Source: CAD feature listing. Evaluate the final solid. Frame: model axes, mm. A direction names the side the tool comes from. Give positions to 0.01 mm unless a question says otherwise; leave off trailing zeros. Order: outer loops, then holes, each group sorted by start corner. A loop starts at its lowest first (then second) coordinate and runs counter-clockwise, first axis right, second up.
from build123d import *

# Parameters (mm, degrees)
SKETCH_1_W          = 5000
SKETCH_1_H          = 1500
EXTRUDE_1_DEPTH     = 30
EXTRUDE_2_DEPTH     = 1500
EXTRUDE_3_REACH     = 5218.234
EXTRUDE_4_REACH     = 5168.168
SKETCH_5_W          = 130
SKETCH_5_H          = 10
FILLET_2_R          = 80
SKETCH_6_R          = 30
CUT_EXTRUDE_1_DEPTH = 1355
SCALE_1_SCALE       = 0.345


with BuildPart() as part:
    # 草图1 → 凸台-拉伸1 (new body)
    with BuildSketch(Plane.XY):
        with Locations((2446.443283418, -722.784179357)):
            Rectangle(SKETCH_1_W, SKETCH_1_H)
    extrude(amount=EXTRUDE_1_DEPTH)

    # 草图3 → 凸台-拉伸2 (add)
    with BuildSketch(Plane(origin=(0, 27.215820643, 0), x_dir=(1, 0, 0), z_dir=(0, 1, 0))):
        Polygon((-53.556716582, 0), (21.443283418, 0), (21.443283418, 200), (-53.556716582, 200), (-53.556716582, 191), (12.443283418, 191), (12.443283418, 9), (-53.556716582, 9), align=None)
        Polygon((4946.443283418, 9), (4946.443283418, 0), (4871.443283418, 0), (4871.443283418, 200), (4946.443283418, 200), (4946.443283418, 191), (4880.443283418, 191), (4880.443283418, 9), align=None)
    extrude(amount=-EXTRUDE_2_DEPTH)

    # 凸台-拉伸3: up to this face of the body (flat: up to its plane)
    extrude_3_end = Plane(part.part.faces().sort_by_distance((-53.556716582, -722.784179357, 10.5))[0])
    # 草图4 → 凸台-拉伸3 (add, up to the picked face)
    with BuildSketch(Plane(origin=(4946.443283418, 0, 0), x_dir=(0, 0, -1), z_dir=(1, 0, 0)), mode=Mode.PRIVATE) as extrude_3_sk1:
        Polygon((200, 27.215820643), (0, 27.215820643), (0, -47.784179357), (9, -47.784179357), (9, 18.215820643), (191, 18.215820643), (191, -47.784179357), (200, -47.784179357), align=None)
    extrude_3_tool1 = split(extrude(extrude_3_sk1.sketch, amount=-EXTRUDE_3_REACH, mode=Mode.PRIVATE), bisect_by=extrude_3_end, keep=Keep.BOTH, mode=Mode.PRIVATE)
    # 草图4 → 凸台-拉伸3 (add, up to the picked face)
    with BuildSketch(Plane(origin=(4946.443283418, 0, 0), x_dir=(0, 0, -1), z_dir=(1, 0, 0)), mode=Mode.PRIVATE) as extrude_3_sk2:
        Polygon((9, -1397.784179357), (0, -1397.784179357), (0, -1472.784179357), (200, -1472.784179357), (200, -1397.784179357), (191, -1397.784179357), (191, -1463.784179357), (9, -1463.784179357), align=None)
    extrude_3_tool2 = split(extrude(extrude_3_sk2.sketch, amount=-EXTRUDE_3_REACH, mode=Mode.PRIVATE), bisect_by=extrude_3_end, keep=Keep.BOTH, mode=Mode.PRIVATE)
    add(extrude_3_tool1.solids().sort_by(Axis((4946.443283, 25.07982, -100), (-1, 0, 0)))[0])
    add(extrude_3_tool2.solids().sort_by(Axis((4946.443283, -1399.92018, -4.5), (-1, 0, 0)))[0])

    # 凸台-拉伸4: up to this face of the body (flat: up to its plane)
    extrude_4_end = Plane(part.part.faces().sort_by_distance((2446.443283418, -722.784179357, 0))[0])
    # 草图5 → 凸台-拉伸4 (add, up to the picked face)
    with BuildSketch(Plane(origin=(0, 0, -200), x_dir=(-1, 0, 0), z_dir=(0, 0, -1)), mode=Mode.PRIVATE) as extrude_4_sk1:
        with Locations((-86.443283418, -52.784179357)):
            Rectangle(SKETCH_5_W, SKETCH_5_H)
    extrude_4_tool1 = split(extrude(extrude_4_sk1.sketch, amount=-EXTRUDE_4_REACH, mode=Mode.PRIVATE), bisect_by=extrude_4_end, keep=Keep.BOTH, mode=Mode.PRIVATE)
    # 草图5 → 凸台-拉伸4 (add, up to the picked face)
    with BuildSketch(Plane(origin=(0, 0, -200), x_dir=(-1, 0, 0), z_dir=(0, 0, -1)), mode=Mode.PRIVATE) as extrude_4_sk2:
        with Locations((-86.443283418, -174.784179357)):
            Rectangle(SKETCH_5_W, SKETCH_5_H)
    extrude_4_tool2 = split(extrude(extrude_4_sk2.sketch, amount=-EXTRUDE_4_REACH, mode=Mode.PRIVATE), bisect_by=extrude_4_end, keep=Keep.BOTH, mode=Mode.PRIVATE)
    # 草图5 → 凸台-拉伸4 (add, up to the picked face)
    with BuildSketch(Plane(origin=(0, 0, -200), x_dir=(-1, 0, 0), z_dir=(0, 0, -1)), mode=Mode.PRIVATE) as extrude_4_sk3:
        with Locations((-86.443283418, -1270.784179357)):
            Rectangle(SKETCH_5_W, SKETCH_5_H)
    extrude_4_tool3 = split(extrude(extrude_4_sk3.sketch, amount=-EXTRUDE_4_REACH, mode=Mode.PRIVATE), bisect_by=extrude_4_end, keep=Keep.BOTH, mode=Mode.PRIVATE)
    # 草图5 → 凸台-拉伸4 (add, up to the picked face)
    with BuildSketch(Plane(origin=(0, 0, -200), x_dir=(-1, 0, 0), z_dir=(0, 0, -1)), mode=Mode.PRIVATE) as extrude_4_sk4:
        with Locations((-86.443283418, -1392.784179357)):
            Rectangle(SKETCH_5_W, SKETCH_5_H)
    extrude_4_tool4 = split(extrude(extrude_4_sk4.sketch, amount=-EXTRUDE_4_REACH, mode=Mode.PRIVATE), bisect_by=extrude_4_end, keep=Keep.BOTH, mode=Mode.PRIVATE)
    add(extrude_4_tool1.solids().sort_by(Axis((86.443283, -52.784179, -200), (0, 0, 1)))[0])
    add(extrude_4_tool2.solids().sort_by(Axis((86.443283, -174.784179, -200), (0, 0, 1)))[0])
    add(extrude_4_tool3.solids().sort_by(Axis((86.443283, -1270.784179, -200), (0, 0, 1)))[0])
    add(extrude_4_tool4.solids().sort_by(Axis((86.443283, -1392.784179, -200), (0, 0, 1)))[0])

    # 圆角2
    # the kernel refuses this fillet: 80 mm, written as the material it takes off along each edge
    with BuildSketch(Plane(origin=(151.443283418, -47.784179357, -200), x_dir=(-1, 0, 0), z_dir=(0, -1, 0))) as fillet_2_piece_1:
        with BuildLine():
            CenterArc((FILLET_2_R, -FILLET_2_R), FILLET_2_R, 90, 90)
            Line((0, -FILLET_2_R), (0, 0))
            Line((0, 0), (FILLET_2_R, 0))
        make_face()
    extrude(amount=210, mode=Mode.SUBTRACT)
    with BuildSketch(Plane(origin=(151.443283418, 30.215820643, -200), x_dir=(-1, 0, 0), z_dir=(0, -1, 0))) as fillet_2_piece_2_section:
        with BuildLine():
            CenterArc((FILLET_2_R, -FILLET_2_R), FILLET_2_R, 90, 90)
            Line((0, -FILLET_2_R), (0, 0))
            Line((0, 0), (FILLET_2_R, 0))
        make_face()
    fillet_2_piece_2 = extrude(amount=410, mode=Mode.PRIVATE)
    fillet_2_piece_2 = split(fillet_2_piece_2, bisect_by=Plane(origin=(123.199877996, -47.784179357, -195.897838893), z_dir=(0, -1, 0)), keep=Keep.TOP, mode=Mode.PRIVATE)
    add(fillet_2_piece_2, mode=Mode.SUBTRACT)
    with BuildSketch(Plane(origin=(151.443283418, -1065.784179357, -200), x_dir=(-1, 0, 0), z_dir=(0, -1, 0))) as fillet_2_piece_3_section:
        with BuildLine():
            CenterArc((FILLET_2_R, -FILLET_2_R), FILLET_2_R, 90, 90)
            Line((0, -FILLET_2_R), (0, 0))
            Line((0, 0), (FILLET_2_R, 0))
        make_face()
    fillet_2_piece_3 = extrude(amount=410, mode=Mode.PRIVATE)
    fillet_2_piece_3 = split(fillet_2_piece_3, bisect_by=Plane(origin=(123.199877996, -1397.784179357, -195.897838893), z_dir=(0, 1, 0)), keep=Keep.TOP, mode=Mode.PRIVATE)
    add(fillet_2_piece_3, mode=Mode.SUBTRACT)
    with BuildSketch(Plane(origin=(151.443283418, -1397.784179357, -200), x_dir=(-1, 0, 0), z_dir=(0, 1, 0))) as fillet_2_piece_4:
        with BuildLine():
            CenterArc((FILLET_2_R, FILLET_2_R), FILLET_2_R, 180, 90)
            Line((0, FILLET_2_R), (0, 0))
            Line((0, 0), (FILLET_2_R, 0))
        make_face()
    extrude(amount=210, mode=Mode.SUBTRACT)

    # 草图6 → 切除-拉伸1 (cut)
    with BuildSketch(Plane(origin=(0, -47.784179357, 0), x_dir=(1, 0, 0), z_dir=(0, 1, 0))):
        with Locations(Location((101.443283418, 120, 0), (0, 0, 270))):
            Circle(SKETCH_6_R)
    extrude(amount=-CUT_EXTRUDE_1_DEPTH, mode=Mode.SUBTRACT)


with BuildPart() as part_1:
    # 缩放比例1: scaled about (0, 0, 0)
    add(part.part.scale(SCALE_1_SCALE))


solid = part_1.part
1) Pull-direction query (X, two-part tool) for faces 1 (the face through (25, -62.026, -35)), 2 (the face through (832, -508.111, -30)), 3 (the face through (-18.477, -267, 0)); classes: +X half, -X half, draft (parallel to the pull), parting line (faces both ways), or undercut.
Checks:
face 1: undercut
face 2: draft
face 3: -X half
2) Section query A-A on x = 785. Output: boundary loops of the cut face in (y, z) (3 decimals), and give its area (3 significant figures).
Checks:
outline: (-508.111, -69) - (-482.236, -69) - (-482.236, -65.895) - (-505.006, -65.895) - (-505.006, -3.105) - (-482.236, -3.105) - (-482.236, 0) - (-16.486, 0) - (-16.486, -3.105) - (6.284, -3.105) - (6.284, -65.895) - (-16.486, -65.895) - (-16.486, -69) - (9.389, -69) - (9.389, 10.35) - (-508.111, 10.35) - close
area: 6,070 mm2
3) First-contact query: pin 1 Ø2 at (y, z) = (-396, -8.5) entering from -X; pin 2 Ø4 at (y, z) = (-439, -21) entering from +X; pin 3 Ø3 at (x, y) = (202.5, -434) entering from -Z. Flat tips, straight axial feed; report the tip coordinate or a pass-through.
Checks:
pin 1: stops at x = 4.29
pin 2: stops at x = 1683.75
pin 3: stops at z = 0
4) Ray query, L1, parallel to X at y = -59.55, z = -41.4; L2, parallel to X at y = -19, z = -41; L3, parallel to Y at x = 1500.5, z = -24. Return the intervals inside material, ascending.
Checks:
L1: x = 4.29 to 24.65, 45.35 to 52.25, 1680.65 to 1683.75
L2: x = 4.29 to 24.66, 45.34 to 52.25, 1680.65 to 1683.75
L3: y = -508.11 to -505.01, 6.28 to 9.39
5) Reachability of faces 4 (the face through (1683.753, -246, -35)), 5 (the face through (25, -482.236, -35)), 6 (the face through (25, -478.786, -35)) from +Z, -Z, +X, -X, +Y, -Y: full face, straight path, thin tool, end or side. Return the list, or none.
Checks:
face 4: +X
face 5: none
face 6: -Z
6) Section query B-B on y = -35.5. Output: boundary loops of the cut face in (x, z) (3 decimals), and give its area (3 significant figures).
Checks:
outline: (-18.477, -69) - (7.398, -69) - (7.398, 0) - (1680.648, 0) - (1680.648, -69) - (1706.523, -69) - (1706.523, -65.895) - (1683.753, -65.895) - (1683.753, -3.105) - (1706.523, -3.105) - (1706.523, 10.35) - (-18.477, 10.35) - (-18.477, -3.105) - (4.293, -3.105) - (4.293, -65.895) - (-18.477, -65.895) - close
area: 18,600 mm2
